Here's the drawing with two shaded views (mm, measured from the low corner). I have some questions. Coordinates: 2 decimals unless noted, no trailing zeros. Loops run counter-clockwise (first coordinate to the right, second up) from the corner with the lowest first, then second, coordinate; pieces in that order, holes last.
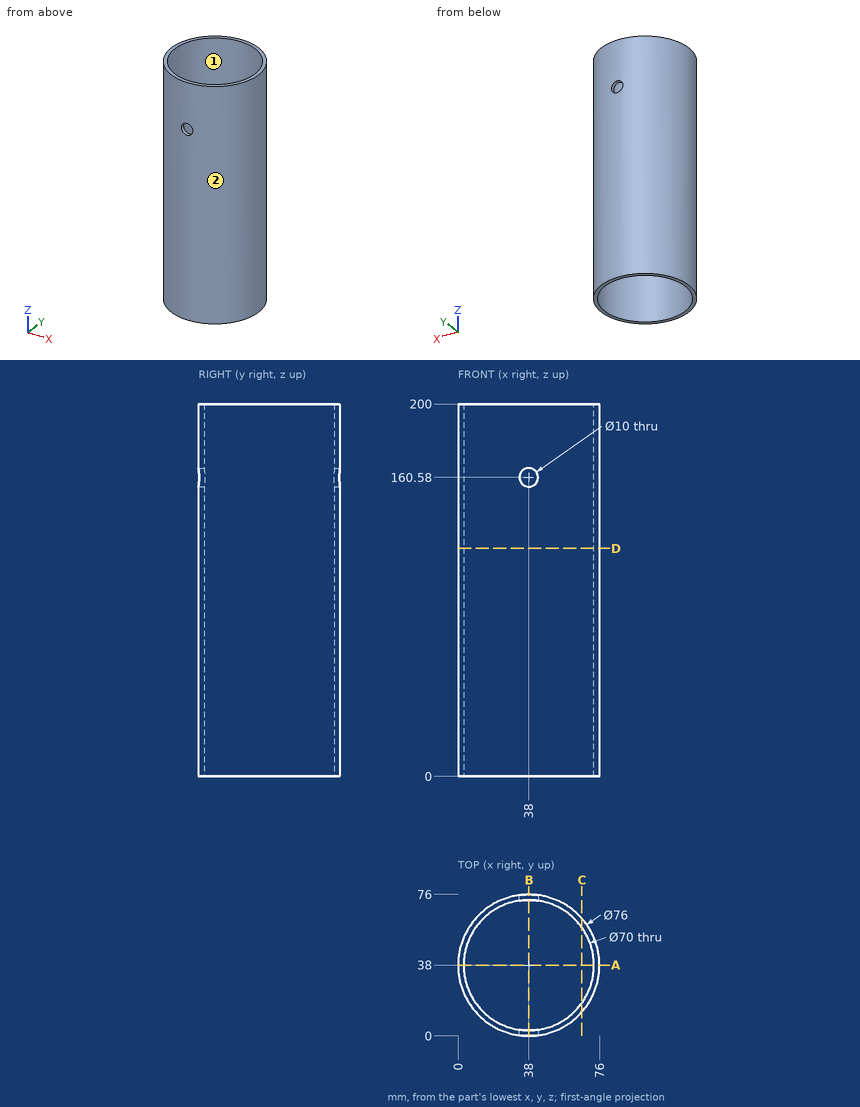
(1) I want a section at D-D on z = 122.5. Write out the boundary of the cut face in (x, y).
Check values:
outline: circle Ø76 at (38, 38); hole circle Ø70 at (38, 38)
(2) If I drill on probe 1 along Y at (x, z) = (37.5, 15); probe 2 along Y at (x, z) = (41, 52); probe 3 along X at (y, z) = (13, 153) (1 decimal), over which ranges is the centre line in solid material (lowest first)?
Check values:
probe 1: y = 0 to 3, 73 to 76
probe 2: y = 0.12 to 3.13, 72.87 to 75.88
probe 3: x = 9.4 to 13.5, 62.5 to 66.6
(3) I want a section at A-A on y = 38. Write out the boundary of the cut face in (x, z), then the cut area to 3 significant figures.
Check values:
outline: (0, 0) - (3, 0) - (3, 200) - (0, 200) - close; (73, 0) - (76, 0) - (76, 200) - (73, 200) - close
area: 1,200 mm2
(4) I want a section at B-B on x = 38. Write out the boundary of the cut face in (y, z).
Check values:
outline: (0, 0) - (3, 0) - (3, 155.58) - (0, 155.58) - close; (0, 165.58) - (3, 165.58) - (3, 200) - (0, 200) - close; (73, 0) - (76, 0) - (76, 155.58) - (73, 155.58) - close; (73, 165.58) - (76, 165.58) - (76, 200) - (73, 200) - close
(5) I want a section at C-C on x = 66.5. Write out the boundary of the cut face in (y, z) (1 decimal), then the cut area to 3 significant figures.
Check values:
outline: (12.9, 0) - (17.7, 0) - (17.7, 200) - (12.9, 200) - close; (58.3, 0) - (63.1, 0) - (63.1, 200) - (58.3, 200) - close
area: 1,930 mm2
(6) If we mould it in two halves opening along X, with no side actions, what happens to the marked faces 1 and 2? For each: released by +X, released by -X, zero draft, split by the parting line, or undercut.
Check values:
face 1: undercut
face 2: split by the parting line
(7) I'm going to push flat-ended pins straight in: pin 1 (10 mm diameter, centred on x = 51, z = 80.5, fed in from +Y); pin 2 (2 mm diameter, centred on x = 33.5, z = 60, fed in from +Y); pin 3 (12 mm diameter, centred on x = 24, z = 52.5, fed in from -Y). Where does each tip first touch, or does it pass through?
Check values:
pin 1: stops at y = 75.15
pin 2: stops at y = 75.84
pin 3: stops at y = 0.85
